```python
from build123d import *

# Parameters (mm, degrees)
ESQUISSE1_R        = 13.5
BOSS_EXTRU_1_DEPTH = 3
ESQUISSE2_R        = 10
BOSS_EXTRU_2_DEPTH = 4
ESQUISSE3_R        = 11.75
BOSS_EXTRU_3_DEPTH = 28
ESQUISSE4_W        = 1.593426019
ESQUISSE4_H        = 0.348561941
BOSS_EXTRU_4_DEPTH = 2.8
CONG_1_R           = 2
CONG_2_R           = 1
CONG_3_R           = 1


with BuildPart() as part:
    # Esquisse1 → Boss.-Extru.1 (new body)
    with BuildSketch(Plane(origin=(0, 0, 0), x_dir=(1, 0, 0), z_dir=(0, 1, 0))):
        with Locations(Location((0, 0, 0), (0, 0, 270))):
            Circle(ESQUISSE1_R)
    extrude(amount=BOSS_EXTRU_1_DEPTH)

    # Esquisse2 → Boss.-Extru.2 (add)
    with BuildSketch(Plane(origin=(0, 3, 0), x_dir=(1, 0, 0), z_dir=(0, 1, 0))):
        with Locations(Location((0, 0, 0), (0, 0, 270))):
            Circle(ESQUISSE2_R)
    extrude(amount=BOSS_EXTRU_2_DEPTH)

    # Esquisse3 → Boss.-Extru.3 (add)
    with BuildSketch(Plane.XZ):
        with Locations(Location((0, 0, 0), (0, 0, 270))):
            Circle(ESQUISSE3_R)
    extrude(amount=BOSS_EXTRU_3_DEPTH)

    # Esquisse4 → Boss.-Extru.4 (add)
    with BuildSketch(Plane.XZ.offset(28)):
        with Locations((-6.369565613, -2.707032561)):
            Rectangle(ESQUISSE4_W, ESQUISSE4_H)
    boss_extru_4 = extrude(amount=BOSS_EXTRU_4_DEPTH)

    # Symétrie1: Boss.-Extru.4 across plane
    add(boss_extru_4.mirror(Plane(origin=(0, 0, 0), x_dir=(0, 0, 1), z_dir=(1, 0, 0))))

    # Congé1
    cong_1_edges = [part.edges().sort_by_distance(p)[0] for p in [
        (0, 7, -10),
    ]]
    fillet(cong_1_edges, radius=CONG_1_R)

    # Congé2
    cong_2_edges = [part.edges().sort_by_distance(p)[0] for p in [
        (0, 3, -13.5),
    ]]
    fillet(cong_2_edges, radius=CONG_2_R)

    # Congé3
    cong_3_edges = [part.edges().sort_by_distance(p)[0] for p in [
        (0, -28, 11.75),
    ]]
    fillet(cong_3_edges, radius=CONG_3_R)


solid = part.part
```
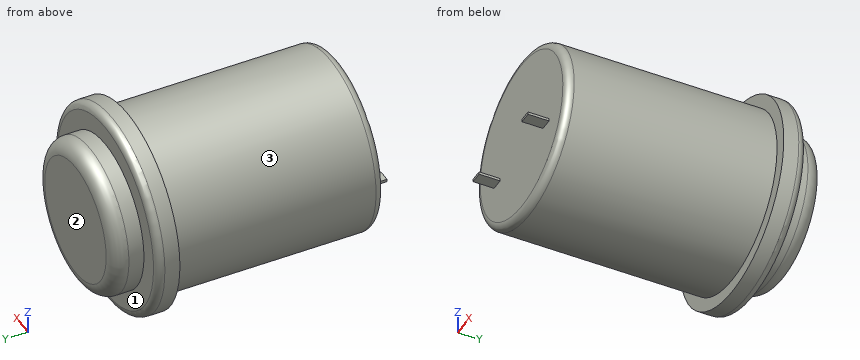
Here's how the part is built. I have some questions about the finished solid (model axes, mm). Face numbers are marked on the shaded views. A direction names the side the tool comes from. Give positions to 0.01 mm unless a question says otherwise; leave off trailing zeros. Order: outer loops, then holes, each group sorted by start corner. A loop starts at its lowest first (then second) coordinate and runs counter-clockwise, first axis right, second up. Notation, with made-up numbers: (-11.5, -16.75) - (42.5, -16.75) arc R21 cw to (42.5, -12.75) - close; hole circle Ø2 at (40.25, 32.5). An arc over 180 degrees is marked (long way). Answer as a JSON object with one key per item and string values. Group by question number.
Item 1: Please list where these lines run through material, in increasing order: probe 1 along Y at (x, z) = (-7.5, 10); probe 2 along Y at (x, z) = (0.75, 10.5); probe 3 along X at (y, z) = (-18, -7.5).
Item 2: If we section it at C-C on y = -10: Please give me the cut outline in (x, z), and give its area (3 significant figures).
Item 3: If we section it at A-A on z = 0: Please give me the cut outline in (x, y), and give its area (3 significant figures).
Item 4: If we section it at B-B on x = 0: Please give me the cut outline in (y, z).
Item 5: Which directions (+Z, -Z, +X, -X, +Y, -Y) give clear straight access to the entire face, cutting with the end or side of a thin tool? Please do the marked faces 1, 2 and 3.
Item 6: For P1, Ø8, axis at y = -5.5, z = 4.5, coming from the +X side; P2, Ø6.5, axis at x = 2, z = 1.5, coming from the -Y side; P3, Ø5, axis at y = -24, z = 8.5, coming from the -X side, each with a flat end and sliding along its axis, tell me the tip position at first contact or that it passes through.
Result set:
{
 "1": {"probe 1": "0 to 3", "probe 2": "-28 to 3", "probe 3": "-9.05 to 9.05"},
 "2": {"outline": "circle Ø23.5 at (0, 0)", "area": "434 mm²"},
 "3": {"outline": "(-13.5, 0) - (-11.75, 0) - (-11.75, -27) arc R1 ccw to (-10.75, -28) - (10.75, -28) arc R1 ccw to (11.75, -27) - (11.75, 0) - (13.5, 0) - (13.5, 2) arc R1 ccw to (12.5, 3) - (10, 3) - (10, 5) arc R2 ccw to (8, 7) - (-8, 7) arc R2 ccw to (-10, 5) - (-10, 3) - (-12.5, 3) arc R1 ccw to (-13.5, 2) - close", "area": "816 mm²"},
 "4": {"outline": "(-28, -10.75) arc R1 ccw to (-27, -11.75) - (0, -11.75) - (0, -13.5) - (2, -13.5) arc R1 ccw to (3, -12.5) - (3, -10) - (5, -10) arc R2 ccw to (7, -8) - (7, 8) arc R2 ccw to (5, 10) - (3, 10) - (3, 12.5) arc R1 ccw to (2, 13.5) - (0, 13.5) - (0, 11.75) - (-27, 11.75) arc R1 ccw to (-28, 10.75) - close"},
 "5": {"face 1": "+Y", "face 2": "+Z, -Z, +X, -X, +Y", "face 3": "-Y"},
 "6": {"P1": "x = 11.74", "P2": "y = -28", "P3": "x = -10.1"}
}
